Can you work these out from the model? Positions are in its coordinate system, mm. Give positions to 0.01 mm unless a question says otherwise; leave off trailing zeros. Loops run counter-clockwise (first coordinate to the right, second up) from the corner with the lowest first, then second, coordinate; pieces in that order, holes last. Notation, with made-up numbers: (-3.75, 78) - (20.25, 78) arc R32 cw to (20.25, 113) - close; hole circle Ø7 at (-28, 87.25). An arc over 180 degrees is marked (long way). Answer as a JSON object with one key per item and string values.
Autodesk Inventor part; units mm, degrees
ref_plane "dia1_XY" through (0, 3.175, 0) normal (1, 0, 0) x (0, 0, -1)
ref_plane "dia1_YZ" through (0, 3.175, 0) normal (0, 0, -1) x (0, 1, 0)
ref_plane "dia1_ZX" through (0, 3.175, 0) normal (0, 1, 0) x (1, 0, 0)
sketch "Sketch_1" plane through (0, 0, 0) normal (0, 0, 1) x (1, 0, 0)
  line L0 (671.5252, 0) -> (0, 0)
  line L1 (0, 0) -> (0, 3.175)
  line L2 (0, 3.175) -> (650.0876, 3.175)
  line L3 (650.0876, 3.175) -> (650.0876, 9.6203)
  line L4 (650.0876, 9.6203) -> (671.5252, 9.6203)
  line L5 (671.5252, 9.6203) -> (671.5252, 0)
  line L6 (671.5252, 0) -> (0, 0)
revolve "Revolution1" add sketch "Sketch_1" angle 360 about axis through (671.5252, 0, 0) along (1, 0, 0)
sketch "Sketch_3" plane through (0, 0, 0) normal (0, 0, 1) x (1, 0, 0)
  line L0 (0, 0) -> (-12.7, 0)
  line L1 (-12.7, 0) -> (-12.7, 2.634)
  line L2 (-12.7, 2.634) -> (-12.159, 3.175)
  line L3 (-12.159, 3.175) -> (0, 3.175)
  line L4 (0, 3.175) -> (0, 0)
  line L5 (0, 0) -> (-12.7, 0)
revolve "Revolution2" add sketch "Sketch_3" angle 360 about axis through (0, 0, 0) along (1, 0, 0)
thread "Thread1"
sketch "Sketch_30" plane through (0, 0, 0) normal (0, 0, 1) x (1, 0, 0)
  line L0 (0, 0) -> (-0.254, 0)
  line L1 (-0.254, 2.921) -> (0, 2.921)
  line L2 (0, 2.921) -> (0, 3.429)
  line L3 (0, 3.429) -> (-0.254, 3.429)
  line L4 (-0.254, 3.429) -> (-0.254, 2.921)
revolve "Revolution3" cut sketch "Sketch_30" angle 360 about axis through (0, 0, 0) along (1, 0, 0)
ref_plane "dia1_XY" through (0, 3.175, 0) normal (1, 0, 0) x (0, 0, -1)
ref_plane "dia1_YZ" through (0, 3.175, 0) normal (0, 0, -1) x (0, 1, 0)
ref_plane "dia1_ZX" through (0, 3.175, 0) normal (0, 1, 0) x (1, 0, 0)
ref_plane "dia12_XY" through (0, 0, 10.9537) normal (1, 0, 0) x (0, 0, -1)
ref_plane "dia12_YZ" through (0, 0, 10.9537) normal (0, 0, -1) x (0, 1, 0)
ref_plane "dia12_ZX" through (0, 0, 10.9537) normal (0, 1, 0) x (1, 0, 0)
ref_plane "dia2_XY" through (0, -3.175, 0) normal (1, 0, 0) x (0, 0, -1)
ref_plane "dia2_YZ" through (0, -3.175, 0) normal (0, 0, -1) x (0, 1, 0)
ref_plane "dia2_ZX" through (0, -3.175, 0) normal (0, 1, 0) x (1, 0, 0)
ref_plane "dia22_XY" through (0, 0, -10.9537) normal (1, 0, 0) x (0, 0, -1)
ref_plane "dia22_YZ" through (0, 0, -10.9537) normal (0, 0, -1) x (0, 1, 0)
ref_plane "dia22_ZX" through (0, 0, -10.9537) normal (0, 1, 0) x (1, 0, 0)
ref_plane "rl1_XY" through (-12.7, 0, 0) normal (1, 0, 0) x (0, 0, -1)
ref_plane "rl1_YZ" through (-12.7, 0, 0) normal (0, 0, -1) x (0, 1, 0)
ref_plane "rl1_ZX" through (-12.7, 0, 0) normal (0, 1, 0) x (1, 0, 0)
ref_plane "rl2_XY" through (0, 0, 0) normal (1, 0, 0) x (0, 0, -1)
ref_plane "rl2_YZ" through (0, 0, 0) normal (0, 0, -1) x (0, 1, 0)
ref_plane "rl2_ZX" through (0, 0, 0) normal (0, 1, 0) x (1, 0, 0)
ref_plane "rod_cp_XY" through (0, 0, 0) normal (1, 0, 0) x (0, 0, -1)
ref_plane "rod_cp_YZ" through (0, 0, 0) normal (0, 0, -1) x (0, 1, 0)
ref_plane "rod_cp_ZX" through (0, 0, 0) normal (0, 1, 0) x (1, 0, 0)
ref_plane "thd1_XY" through (-12.7, 3.175, 0) normal (1, 0, 0) x (0, 0, -1)
ref_plane "thd1_YZ" through (-12.7, 3.175, 0) normal (0, 0, -1) x (0, 1, 0)
ref_plane "thd1_ZX" through (-12.7, 3.175, 0) normal (0, 1, 0) x (1, 0, 0)
ref_plane "thd2_XY" through (-12.7, -3.175, 0) normal (1, 0, 0) x (0, 0, -1)
ref_plane "thd2_YZ" through (-12.7, -3.175, 0) normal (0, 0, -1) x (0, 1, 0)
ref_plane "thd2_ZX" through (-12.7, -3.175, 0) normal (0, 1, 0) x (1, 0, 0)
ref_plane "to_rod_clevis_XY" through (-16.764, 0, 0) normal (1, 0, 0) x (0, 0, -1)
ref_plane "to_rod_clevis_YZ" through (-16.764, 0, 0) normal (0, 0, -1) x (0, 1, 0)
ref_plane "to_rod_clevis_ZX" through (-16.764, 0, 0) normal (0, 1, 0) x (1, 0, 0)
properties part number "SR-0424-DPY0000_rod"
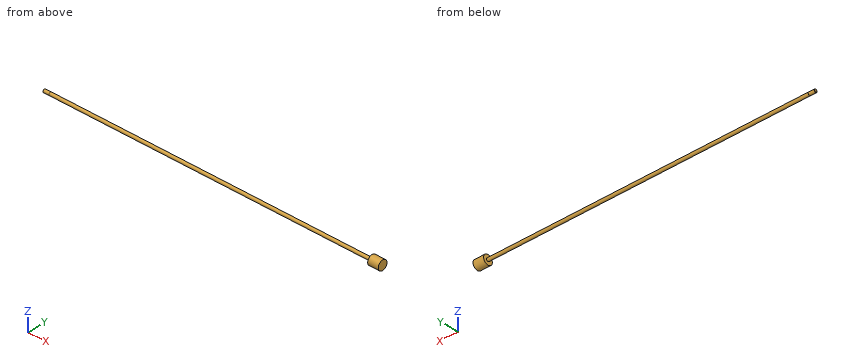
1) Imagine slicing it at A-A on x = 279. Write out the boundary of the cut face in (y, z) (3 decimals), and give its area (3 significant figures).
Check sheet entries:
{"outline": "circle Ø6.35 at (0, 0)", "area": "31.7 mm2"}
2) I need wall thicknesses on L1, parallel to X at y = -6.25, z = -3; L2, parallel to Z at x = 563, y = 0 (3 decimals); L3, parallel to Z at x = 473, y = 0.75. Which ranges of each line are inside material? Lowest first, please.
Check sheet entries:
{"L1": "650.09 to 671.53", "L2": "-3.175 to 3.175", "L3": "-3.09 to 3.09"}
3) I'm going to push flat-ended pins straight in: P1, Ø3, axis at y = -5, z = -4.5, coming from the -X side; P2, Ø5, axis at x = 221, y = 4, coming from the +Z side; P3, Ø8, axis at x = 559.5, z = 2, coming from the -Y side (3 decimals). Where does each tip first touch, or does it pass through?
Check sheet entries:
{"P1": "x = 650.09", "P2": "z = 2.8", "P3": "y = -3.175"}
